from build123d import *

# Parameters (mm, degrees)
CROQUIS1_W              = 40.6
CROQUIS1_H              = 19.5
EXTRUIR1_DEPTH          = 21.55
CROQUIS2_R              = 2.95
EXTRUIR2_DEPTH          = 5
CROQUIS4_W              = 7.8
CROQUIS4_H              = 17.9
CROQUIS4_R              = 1.95
SALIENTE_EXTRUIR1_DEPTH = 1.5


with BuildPart() as part:
    # Croquis1 → Extruir1 (new, symmetric)
    with BuildSketch(Plane(origin=(0, 0, 0), x_dir=(1, 0, 0), z_dir=(0, 1, 0))):
        with Locations((-0.05, -0.1)):
            Rectangle(CROQUIS1_W, CROQUIS1_H)
    extrude(amount=EXTRUIR1_DEPTH, both=True)

    # Croquis2 → Extruir2 (add)
    with BuildSketch(Plane(origin=(0, 21.55, 0), x_dir=(1, 0, 0), z_dir=(0, 1, 0))):
        with Locations(Location((10.650489708, -0.00303525, 0), (0, 0, 90))):
            Circle(CROQUIS2_R)
    extrude(amount=EXTRUIR2_DEPTH)

    # Croquis4 → Saliente-Extruir1 (add, symmetric)
    # profile 1 of 2: a face of its own
    with BuildSketch(Plane(origin=(0, 0, 0), x_dir=(-1, 0, 0), z_dir=(0, 1, 0))):
        with Locations((-24.15, 0)):
            Rectangle(CROQUIS4_W, CROQUIS4_H)
        with Locations(Location((-24.15, -4.95, 0), (0, 0, 90))):
            Circle(CROQUIS4_R, mode=Mode.SUBTRACT)
        with Locations(Location((-24.15, 4.95, 0), (0, 0, 270))):
            Circle(CROQUIS4_R, mode=Mode.SUBTRACT)
    # profile 2 of 2: a face of its own
    with BuildSketch(Plane(origin=(0, 0, 0), x_dir=(-1, 0, 0), z_dir=(0, 1, 0))):
        with Locations((24.15, 0)):
            Rectangle(CROQUIS4_W, CROQUIS4_H)
        with Locations(Location((24.15, -4.95, 0), (0, 0, 270))):
            Circle(CROQUIS4_R, mode=Mode.SUBTRACT)
        with Locations(Location((24.15, 4.95, 0), (0, 0, 90))):
            Circle(CROQUIS4_R, mode=Mode.SUBTRACT)
    extrude(amount=SALIENTE_EXTRUIR1_DEPTH, both=True)


solid = part.part
The listing builds one solid part. Answer for the finished solid, in the listing's coordinates (mm). A direction names the side the tool comes from. Give positions to 0.01 mm unless a question says otherwise; leave off trailing zeros. Order: outer loops, then holes, each group sorted by start corner. A loop starts at its lowest first (then second) coordinate and runs counter-clockwise, first axis right, second up. Notation, with made-up numbers: (47, 15.25) - (88, 15.25) arc R8 cw to (88, 23.25) - close; hole circle Ø1 at (55, 17.25). An arc over 180 degrees is marked (long way). Answer as CSV lines item,"result".
Q1. Each of these flat-tipped pins is pushed along its axis until it touches: pin 1 Ø6 at (x, z) = (24.5, -1) entering from -Y; pin 2 Ø6 at (y, z) = (21.5, -1) entering from +X; pin 3 Ø3 at (y, z) = (-10.5, 1.5) entering from -X. Where does it stop, or does it pass through?
Answer key:
pin 1,"stops at y = -1.5"
pin 2,"stops at x = 20.25"
pin 3,"stops at x = -20.35"
Q2. A cutting plane is placed at C-C, the plane z = -4.5. Determine the outline of the cut face in (x, y).
Answer key:
outline,"(-28.05, -1.5) - (-26.05, -1.5) - (-26.05, 1.5) - (-28.05, 1.5) - close; (-22.25, -1.5) - (-20.35, -1.5) - (-20.35, -21.55) - (20.25, -21.55) - (20.25, -1.5) - (22.25, -1.5) - (22.25, 1.5) - (20.25, 1.5) - (20.25, 21.55) - (-20.35, 21.55) - (-20.35, 1.5) - (-22.25, 1.5) - close; (26.05, -1.5) - (28.05, -1.5) - (28.05, 1.5) - (26.05, 1.5) - close"
Q3. A cutting plane is placed at B-B, the plane z = 4.95. Determine the outline of the cut face in (x, y).
Answer key:
outline,"(-28.05, -1.5) - (-26.1, -1.5) - (-26.1, 1.5) - (-28.05, 1.5) - close; (-22.2, -1.5) - (-20.35, -1.5) - (-20.35, -21.55) - (20.25, -21.55) - (20.25, -1.5) - (22.2, -1.5) - (22.2, 1.5) - (20.25, 1.5) - (20.25, 21.55) - (-20.35, 21.55) - (-20.35, 1.5) - (-22.2, 1.5) - close; (26.1, -1.5) - (28.05, -1.5) - (28.05, 1.5) - (26.1, 1.5) - close"
Q4. Straight lines are drawn through the part: L1, parallel to X at y = -0.4, z = -4.95; L2, parallel to Z at x = -24, y = 0; L3, parallel to Y at x = 6, z = -6.25. For each, find the intervals that lie inside material, in ascending order.
Answer key:
L1,"x = -28.05 to -26.1, -22.2 to 22.2, 26.1 to 28.05"
L2,"z = -8.95 to -6.89, -3.01 to 3.01, 6.89 to 8.95"
L3,"y = -21.55 to 21.55"
Q5. Determine the mould class of faces 5 (the face through (0, 0, -9.65)), 6 (the face through (25.337, -0.021, 6.497)), 7 (the face through (7.726, 24.015, 0.387)) for opening direction X: pulls with the +X half, pulls with the -X half, needs draft (parallel to the pull), parting line crosses it, or undercut.
Answer key:
face 5,"needs draft"
face 6,"undercut"
face 7,"parting line crosses it"
Q6. A cutting plane is placed at A-A, the plane x = -24.15. Determine the outline of the cut face in (y, z).
Answer key:
outline,"(-1.5, -8.95) - (1.5, -8.95) - (1.5, -6.9) - (-1.5, -6.9) - close; (-1.5, -3) - (1.5, -3) - (1.5, 3) - (-1.5, 3) - close; (-1.5, 6.9) - (1.5, 6.9) - (1.5, 8.95) - (-1.5, 8.95) - close"
Q7. Which of the six approach directions +Z, -Z, +X, -X, +Y, -Y give full straight-line access (tool end or side, diameter ignored) to faces 1 (the face through (-24, 1.5, 0)), 2 (the face through (-24, -1.5, 0)), 3 (the face through (24, 0, 8.95)), 4 (the face through (24, -1.5, 0))?
Answer key:
face 1,"+Z, -Z, -X, +Y"
face 2,"+Z, -Z, -X, -Y"
face 3,"+Z, +X, +Y, -Y"
face 4,"+Z, -Z, +X, -Y"
Q8. A cutting plane is placed at D-D, the plane y = -14. Determine the outline of the cut face in (x, z).
Answer key:
outline,"(-20.35, -9.65) - (20.25, -9.65) - (20.25, 9.85) - (-20.35, 9.85) - close"
